```python
from build123d import *

# Parameters (mm, degrees)
SKETCH1_R                = 37.5
SKETCH1_R_2              = 12.5
BOSS_EXTRUDE1_DEPTH      = 10
SKETCH2_R                = 12.5
BOSS_EXTRUDE2_DEPTH      = 40
SKETCH3_R                = 37.5
SKETCH3_R_2              = 12.5
BOSS_EXTRUDE3_DEPTH      = 10
SKETCH4_W                = 40
SKETCH4_H                = 55.901699438
BOSS_EXTRUDE4_DEPTH      = 35
SKETCH5_R                = 20
BOSS_EXTRUDE5_DEPTH      = 55
SKETCH6_W                = 40
SKETCH6_H                = 45.901699438
BOSS_EXTRUDE6_DEPTH      = 45
BOSS_EXTRUDE7_DEPTH      = 45
BOSS_EXTRUDE7_DEPTH_BACK = 200
SKETCH7_R                = 17.5


with BuildPart() as part:
    # Sketch1 → Boss-Extrude1 (new body)
    with BuildSketch(Plane.XY):
        Circle(SKETCH1_R)
        Circle(SKETCH1_R_2, mode=Mode.SUBTRACT)
    extrude(amount=BOSS_EXTRUDE1_DEPTH)

    # Sketch2 → Boss-Extrude2 (add)
    with BuildSketch(Plane.XY.offset(10)):
        with BuildLine():
            Line((25, 27.950849719), (25, -27.950849719))
            ThreePointArc((25, -27.950849719), (-37.5, 0), (25, 27.950849719))
        make_face()
        Circle(SKETCH2_R, mode=Mode.SUBTRACT)
    extrude(amount=BOSS_EXTRUDE2_DEPTH)

    # Sketch3 → Boss-Extrude3 (add)
    with BuildSketch(Plane.XY.offset(50)):
        Circle(SKETCH3_R)
        Circle(SKETCH3_R_2, mode=Mode.SUBTRACT)
    extrude(amount=BOSS_EXTRUDE3_DEPTH)

    # Sketch4 → Boss-Extrude4 (add)
    with BuildSketch(Plane(origin=(25, 0, 0), x_dir=(0, 0, -1), z_dir=(1, 0, 0))):
        with Locations((-30, 0)):
            Rectangle(SKETCH4_W, SKETCH4_H)
    extrude(amount=BOSS_EXTRUDE4_DEPTH)

    # Sketch5 → Boss-Extrude5 (add)
    with BuildSketch(Plane(origin=(60, 0, 0), x_dir=(0, 0, -1), z_dir=(1, 0, 0))):
        with Locations((-30, 0)):
            Circle(SKETCH5_R)
    extrude(amount=BOSS_EXTRUDE5_DEPTH)

    # Sketch6 → Boss-Extrude6 (add)
    with BuildSketch(Plane(origin=(115, 0, 0), x_dir=(0, 0, -1), z_dir=(1, 0, 0))):
        with Locations((-30, 0)):
            Rectangle(SKETCH6_W, SKETCH6_H)
    extrude(amount=BOSS_EXTRUDE6_DEPTH)

    # Sketch7 → Boss-Extrude7 (add, two sides: drawn at the far end of the back side and taken through both)
    with BuildSketch(Plane(origin=(0, 22.950849719, 0), x_dir=(1, 0, 0), z_dir=(0, 1, 0)).offset(-BOSS_EXTRUDE7_DEPTH_BACK)):
        with Locations(Location((137.5, -30, 0), (0, 0, 180))):
            Circle(SKETCH7_R)
    extrude(amount=BOSS_EXTRUDE7_DEPTH + BOSS_EXTRUDE7_DEPTH_BACK)


solid = part.part
```
Can you work these out from the model? Positions are in its coordinate system, mm. A direction names the side the tool comes from. Round coordinates to 2 decimals unless told otherwise and drop trailing zeros. Loops run counter-clockwise (first coordinate to the right, second up) from the corner with the lowest first, then second, coordinate; pieces in that order, holes last.
Item 1: Which directions (+Z, -Z, +X, -X, +Y, -Y) give clear straight access to the entire face, cutting with the end or side of a thin tool? Please do faces 5 (the flat face through (137, 0, 50)), 6 (the flat face through (42, -27.951, 30)), 7 (the flat face through (115, 21, 30)), 8 (the cylindrical face through (87.115, 6.007, 10.924)), 9 (the flat face through (60, -23, 30)).
Item 2: Will these pins go through, and if not, where does the flat tip stop? pin 1 Ø1.5 at (y, z) = (-138.5, 26.5) entering from -X; pin 2 Ø12 at (x, z) = (79, 39.5) entering from +Y; pin 3 Ø22.5 at (x, y) = (135.5, 0.5) entering from -Z.
Item 3: Suppose I cut it at C-C, the plane y = 7. Write out the boundary of the cut face in (x, z) (3 decimals), then the cut area to 3 significant figures.
Item 4: If we mould it in two halves opening along X, with no side actions, what happens to faces 1 (the flat face through (122, 22.951, 21)), 2 (the cylindrical face through (128.092, 45.136, 44.756)), 3 (the flat face through (46, 0, 50)), 4 (the flat face through (160, 0, 30))? For each: +X half, -X half, draft (parallel to the pull), parting line (faces both ways), or undercut.
Item 5: Suppose I cut it at B-B, the plane z = 30. Write out the boundary of the cut face in (x, y).
Item 6: Suppose I cut it at A-A, the plane x = 0. Write out the boundary of the cut face in (y, z), then the cut area to 3 significant figures.
Item 7: Please list where these lines run through material, in increasing order: L1, parallel to Y at x = 0, z = 26; L2, parallel to Y at x = 41.5, z = 36; L3, parallel to Y at x = -1.5, z = 54.
Item 8: Suppose I cut it at D-D, the plane x = 137.5. Write out the boundary of the cut face in (y, z).
Reported:
1. face 5: +Z, +X, +Y, -Y
1. face 6: +Z, -Z, -Y
1. face 7: +Y
1. face 8: none
1. face 9: -Y
2. pin 1: stops at x = 120.22
2. pin 2: stops at y = 19.69
2. pin 3: stops at z = 10
3. outline: (-36.841, 0) - (-10.356, 0) - (-10.356, 60) - (-36.841, 60) - close; (10.356, 0) - (36.841, 0) - (36.841, 10) - (60, 10) - (60, 11.265) - (115, 11.265) - (115, 10) - (160, 10) - (160, 50) - (115, 50) - (115, 48.735) - (60, 48.735) - (60, 50) - (36.841, 50) - (36.841, 60) - (10.356, 60) - close
3. area: 7,970 mm2
4. face 1: undercut
4. face 2: undercut
4. face 3: draft
4. face 4: +X half
5. outline: (25, -27.95) - (60, -27.95) - (60, -20) - (115, -20) - (115, -22.95) - (120, -22.95) - (120, -177.05) - (155, -177.05) - (155, -22.95) - (160, -22.95) - (160, 22.95) - (155, 22.95) - (155, 67.95) - (120, 67.95) - (120, 22.95) - (115, 22.95) - (115, 20) - (60, 20) - (60, 27.95) - (25, 27.95) arc R37.5 ccw (long way) to start; hole circle Ø25 at (0, 0)
6. outline: (-37.5, 0) - (-12.5, 0) - (-12.5, 60) - (-37.5, 60) - close; (12.5, 0) - (37.5, 0) - (37.5, 60) - (12.5, 60) - close
6. area: 3,000 mm2
7. L1: y = -37.5 to -12.5, 12.5 to 37.5
7. L2: y = -27.95 to 27.95
7. L3: y = -37.47 to -12.41, 12.41 to 37.47
8. outline: (-177.05, 12.5) - (-22.95, 12.5) - (-22.95, 10) - (22.95, 10) - (22.95, 12.5) - (67.95, 12.5) - (67.95, 47.5) - (22.95, 47.5) - (22.95, 50) - (-22.95, 50) - (-22.95, 47.5) - (-177.05, 47.5) - close
